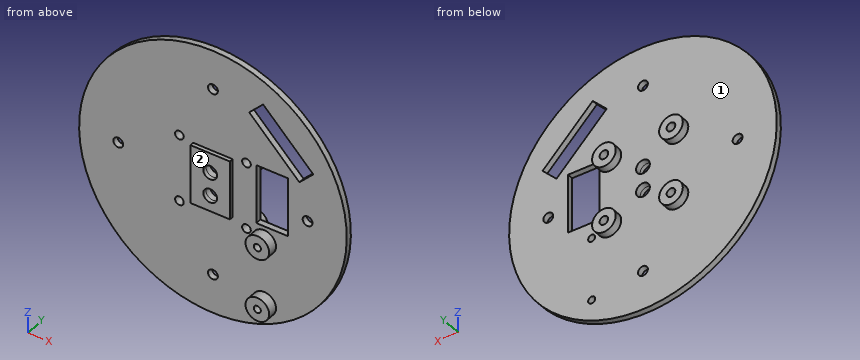
from build123d import *
from build123d.topology import SkipClean

# Parameters (mm, degrees)
SKETCH_1_R      = 33.929985128
SKETCH_1_R_2    = 1.25
SKETCH_1_R_3    = 1.1
SKETCH_1_R_4    = 1.75
SKETCH_1_R_5    = 0.9
SKETCH_1_W      = 8
SKETCH_1_H      = 15
EXTRUDE_1_DEPTH = 1.5
SKETCH_2_R      = 3
SKETCH_2_R_2    = 1.1
EXTRUDE_2_DEPTH = 2
EXTRUDE_START   = 1
SKETCH_3_W      = 10
SKETCH_3_H      = 15
SKETCH_3_R      = 1.75
EXTRUDE_3_DEPTH = 1
EXTRUDE_START_2 = 2.5
SKETCH_5_R      = 3
SKETCH_5_R_2    = 0.9
EXTRUDE_5_DEPTH = 2.5


with BuildPart() as part:
    # 草图1 → 凸台-拉伸1 (new body)
    with BuildSketch(Plane(origin=(0, 0, 0), x_dir=(1, 0, 0), z_dir=(0, 1, 0))):
        with Locations(Location((0, 0, 0), (0, 0, 270))):
            Circle(SKETCH_1_R)
        with Locations(Location((0, 24, 0), (0, 0, 270))):
            Circle(SKETCH_1_R_2, mode=Mode.SUBTRACT)
        with Locations(Location((24, 0, 0), (0, 0, 270))):
            Circle(SKETCH_1_R_2, mode=Mode.SUBTRACT)
        with Locations(Location((0, -24, 0), (0, 0, 270))):
            Circle(SKETCH_1_R_2, mode=Mode.SUBTRACT)
        with Locations(Location((-24, 0, 0), (0, 0, 270))):
            Circle(SKETCH_1_R_2, mode=Mode.SUBTRACT)
        with Locations(Location((8.5, 8.5, 0), (0, 0, 270))):
            Circle(SKETCH_1_R_3, mode=Mode.SUBTRACT)
        with Locations(Location((-8.5, 8.5, 0), (0, 0, 90))):
            Circle(SKETCH_1_R_3, mode=Mode.SUBTRACT)
        with Locations(Location((8.5, -8.5, 0), (0, 0, 90))):
            Circle(SKETCH_1_R_3, mode=Mode.SUBTRACT)
        with Locations(Location((-8.5, -8.5, 0), (0, 0, 270))):
            Circle(SKETCH_1_R_3, mode=Mode.SUBTRACT)
        with Locations(Location((0, 3, 0), (0, 0, 270))):
            Circle(SKETCH_1_R_4, mode=Mode.SUBTRACT)
        with Locations(Location((0, -3, 0), (0, 0, 270))):
            Circle(SKETCH_1_R_4, mode=Mode.SUBTRACT)
        with Locations(Location((13, 10, 0), (0, 0, 270))):
            Circle(SKETCH_1_R_5, mode=Mode.SUBTRACT)
        with Locations(Location((13, 26, 0), (0, 0, 90))):
            Circle(SKETCH_1_R_5, mode=Mode.SUBTRACT)
        Polygon((21.920310217, -9.192388155), (9.192388155, -21.920310217), (12.727922061, -25.455844123), (25.455844123, -12.727922061), align=None, mode=Mode.SUBTRACT)
        with Locations((15, -1.5)):
            Rectangle(SKETCH_1_W, SKETCH_1_H, mode=Mode.SUBTRACT)
    extrude(amount=EXTRUDE_1_DEPTH)

    # 草图2 → 凸台-拉伸2 (add)
    # profile 1 of 4: a face of its own
    with BuildSketch(Plane(origin=(0, 1.5, 0), x_dir=(1, 0, 0), z_dir=(0, 1, 0))):
        with Locations(Location((-8.5, 8.5, 0), (0, 0, 270))):
            Circle(SKETCH_2_R)
        with Locations(Location((-8.5, 8.5, 0), (0, 0, 90))):
            Circle(SKETCH_2_R_2, mode=Mode.SUBTRACT)
    # profile 2 of 4: a face of its own
    with BuildSketch(Plane(origin=(0, 1.5, 0), x_dir=(1, 0, 0), z_dir=(0, 1, 0))):
        with Locations(Location((8.5, 8.5, 0), (0, 0, 270))):
            Circle(SKETCH_2_R)
        with Locations(Location((8.5, 8.5, 0), (0, 0, 270))):
            Circle(SKETCH_2_R_2, mode=Mode.SUBTRACT)
    # profile 3 of 4: a face of its own
    with BuildSketch(Plane(origin=(0, 1.5, 0), x_dir=(1, 0, 0), z_dir=(0, 1, 0))):
        with Locations(Location((8.5, -8.5, 0), (0, 0, 33.557309762))):
            Circle(SKETCH_2_R)
        with Locations(Location((8.5, -8.5, 0), (0, 0, 90))):
            Circle(SKETCH_2_R_2, mode=Mode.SUBTRACT)
    # profile 4 of 4: a face of its own
    with BuildSketch(Plane(origin=(0, 1.5, 0), x_dir=(1, 0, 0), z_dir=(0, 1, 0))):
        with Locations(Location((-8.5, -8.5, 0), (0, 0, 270))):
            Circle(SKETCH_2_R)
        with Locations(Location((-8.5, -8.5, 0), (0, 0, 270))):
            Circle(SKETCH_2_R_2, mode=Mode.SUBTRACT)
    extrude(amount=EXTRUDE_2_DEPTH)

    # 草图3 → 凸台-拉伸3 (add)
    with SkipClean():  # the faces are left unmerged after this step: merging them gives an invalid solid
        with BuildSketch(Plane.XZ.offset(EXTRUDE_START)):
            with Locations((0, 0.5)):
                Rectangle(SKETCH_3_W, SKETCH_3_H)
            with Locations(Location((0, 3, 0), (0, 0, 270))):
                Circle(SKETCH_3_R, mode=Mode.SUBTRACT)
            with Locations(Location((0, -3, 0), (0, 0, 270))):
                Circle(SKETCH_3_R, mode=Mode.SUBTRACT)
        extrude(amount=-EXTRUDE_3_DEPTH)

    # 草图5 → 凸台-拉伸5 (add)
    # profile 1 of 2: a face of its own
    with SkipClean():  # the faces are left unmerged after this step: merging them gives an invalid solid
        with BuildSketch(Plane.XZ.offset(EXTRUDE_START_2)):
            with Locations(Location((13, -26, 0), (0, 0, 90))):
                Circle(SKETCH_5_R)
            with Locations(Location((13, -26, 0), (0, 0, 270))):
                Circle(SKETCH_5_R_2, mode=Mode.SUBTRACT)
        # profile 2 of 2: a face of its own
        with BuildSketch(Plane.XZ.offset(EXTRUDE_START_2)):
            with Locations(Location((13, -10, 0), (0, 0, 90))):
                Circle(SKETCH_5_R)
            with Locations(Location((13, -10, 0), (0, 0, 270))):
                Circle(SKETCH_5_R_2, mode=Mode.SUBTRACT)
        extrude(amount=-EXTRUDE_5_DEPTH)


solid = part.part
Source: CAD feature listing. Evaluate the final solid. Frame: model axes, mm. Face numbers are marked on the shaded views. A direction names the side the tool comes from. Round coordinates to 2 decimals unless told otherwise and drop trailing zeros. Loops run counter-clockwise (first coordinate to the right, second up) from the corner with the lowest first, then second, coordinate; pieces in that order, holes last. Notation, with made-up numbers: (0.25, -13) - (38.25, -13) arc R15 cw to (38.25, 13) - close; hole circle Ø10 at (-38, 20). An arc over 180 degrees is marked (long way). Write item = value, one per line. Start each with the question number.
Item 1: Section query D-D on x = -8.5. Output: boundary loops of the cut face in (y, z).
Item 2: Reachability of the marked faces 1 and 2 from +Z, -Z, +X, -X, +Y, -Y: full face, straight path, thin tool, end or side. Return the list, or none.
Item 3: Section query C-C on z = -24. Output: boundary loops of the cut face in (x, y).
Item 4: Section query B-B on x = -24. Output: boundary loops of the cut face in (y, z), plus the area to 3 significant figures.
Item 5: Section query A-A on z = 0. Output: boundary loops of the cut face in (x, y).
Item 6: Material intervals for line 1 (X direction, y = -1.2, z = -10); line 2 (X direction, y = 0.75, z = 25); line 3 (X direction, y = 0.2, z = 1), sorted ascending.
Item 7: First-contact query: pin 1 Ø4 at (x, z) = (0, 3) entering from +Y; pin 2 Ø2.5 at (x, z) = (-8.5, -8.5) entering from -Y; pin 3 Ø4 at (x, z) = (0, -3) entering from -Y. Flat tips, straight axial feed; report the tip coordinate or a pass-through.
Results list:
q1.outline = (0, -32.85) - (1.5, -32.85) - (1.5, -11.5) - (3.5, -11.5) - (3.5, -9.6) - (0, -9.6) - close; (0, -7.4) - (3.5, -7.4) - (3.5, -5.5) - (1.5, -5.5) - (1.5, 5.5) - (3.5, 5.5) - (3.5, 7.4) - (0, 7.4) - close; (0, 9.6) - (3.5, 9.6) - (3.5, 11.5) - (1.5, 11.5) - (1.5, 32.85) - (0, 32.85) - close
q2.face_1 = +Y
q2.face_2 = +Z, -Z, +X, -X, -Y
q3.outline = (-23.98, 0) - (-1.25, 0) - (-1.25, 1.5) - (-23.98, 1.5) - close; (1.25, 0) - (10.76, 0) - (10.76, -2.5) - (15.24, -2.5) - (15.24, 0) - (23.98, 0) - (23.98, 1.5) - (1.25, 1.5) - close
q4.outline = (0, -23.98) - (1.5, -23.98) - (1.5, -1.25) - (0, -1.25) - close; (0, 1.25) - (1.5, 1.25) - (1.5, 23.98) - (0, 23.98) - close
q4.area = 68.2 mm²
q5.outline = (-33.93, 0) - (-25.25, 0) - (-25.25, 1.5) - (-33.93, 1.5) - close; (-22.75, 0) - (-5, 0) - (-5, -1) - (5, -1) - (5, 0) - (11, 0) - (11, 1.5) - (-22.75, 1.5) - close; (19, 0) - (22.75, 0) - (22.75, 1.5) - (19, 1.5) - close; (25.25, 0) - (33.93, 0) - (33.93, 1.5) - (25.25, 1.5) - close
q6.line_1 = 10 to 12.1, 13.9 to 16
q6.line_2 = -22.94 to -0.75, 0.75 to 12.27, 13.18 to 22.94
q6.line_3 = -33.92 to -24.75, -23.25 to 11, 19 to 23.25, 24.75 to 33.92
q7.pin_1 = 1.5
q7.pin_2 = 0
q7.pin_3 = -1
